Autodesk Inventor part; units mm, degrees
ref_plane "YZ Plane" through (0, 0, 0) normal (1, 0, 0) x (0, 1, 0)
ref_plane "XZ Plane" through (0, 0, 0) normal (0, 1, 0) x (-1, 0, 0)
ref_plane "XY Plane" through (0, 0, 0) normal (0, 0, 1) x (1, 0, 0)
sketch "Esquisse1" plane through (0, 0, 0) normal (0, 0, 1) x (1, 0, 0)
  line L0 (-367.5, -182.5) -> (367.5, -182.5)
  line L1 (367.5, -182.5) -> (367.5, 182.5)
  line L2 (367.5, 182.5) -> (-367.5, 182.5)
  line L3 (-367.5, 182.5) -> (-367.5, -182.5)
  line L4 (-367.5, -182.5) -> (367.5, 182.5) construction
  line L5 (-355, -170) -> (355, -170)
  line L6 (355, -170) -> (355, 170)
  line L7 (355, 170) -> (-355, 170)
  line L8 (-355, 170) -> (-355, -170)
  line L9 (-355, -170) -> (355, 170) construction
  circle A0 centre (-352.5, 167.5) radius 2.5
  circle A1 centre (-352.5, -167.5) radius 2.5
  circle A2 centre (352.5, -167.5) radius 2.5
  circle A3 centre (352.5, 167.5) radius 2.5
  line L10 (-17.5, -40.5) -> (34.5, -40.5)
  line L11 (54.5, -60.5) -> (54.5, -112.5)
  line L12 (34.5, -132.5) -> (-17.5, -132.5)
  line L13 (-37.5, -112.5) -> (-37.5, -60.5)
  line L14 (-37.5, -40.5) -> (54.5, -132.5) construction
  line L15 (54.5, -40.5) -> (-37.5, -132.5) construction
  line L16 (-17.5, -40.5) -> (-37.5, -60.5)
  line L17 (-37.5, -112.5) -> (-17.5, -132.5)
  line L18 (34.5, -132.5) -> (54.5, -112.5)
  line L19 (54.5, -60.5) -> (34.5, -40.5)
  circle A4 centre (-32.75, -45.25) radius 2.2
  circle A5 centre (49.75, -45.25) radius 2.2
  circle A6 centre (49.75, -127.75) radius 2.2
  circle A7 centre (-32.75, -127.75) radius 2.2
  point P0 (0, 0)
  point P1 (-355, -167.5)
  point P2 (-352.5, -170)
  point P3 (352.5, -170)
  point P4 (355, -167.5)
  point P5 (355, 167.5)
  point P6 (352.5, 170)
  point P7 (-355, 167.5)
  point P8 (-352.5, 170)
  point P9 (8.5, -86.5)
  dimension "d0" = 735
  dimension "d1" = 365
  dimension "d2" = 12.5
  dimension "d3" = 12.5
  dimension "d4" = 5
  dimension "d7" = 5
  dimension "d8" = 5
  dimension "d9" = 5
  dimension "d36" = 92
  dimension "d37" = 92
  dimension "d38" = 50
  dimension "d39" = 313
  dimension "d48" = 20
  dimension "d49" = 20
  dimension "d50" = 20
  dimension "d51" = 20
  dimension "d52" = 20
  dimension "d53" = 20
  dimension "d54" = 20
  dimension "d55" = 20
  dimension "d57" = 4.4
  dimension "d58" = 4.4
  dimension "d59" = 4.4
  dimension "d60" = 4.4
  dimension "d61" = 4.75
  dimension "d62" = 4.75
extrude "Extrusion1" add sketch "Esquisse1" along normal blind 2 contours L3 L2 L1 L0 | L8 A1 L5 | A1 L8 A0 L7 A3 L6 A2 L5 | A2 L6 L5 | L8 L7 A0 | A3 L7 L6
properties part number "PlaqueVentilo"
The listing builds one solid part. Answer for the finished solid, in the listing's coordinates (mm). A direction names the side the tool comes from. Round coordinates to 2 decimals unless told otherwise and drop trailing zeros. Loops run counter-clockwise (first coordinate to the right, second up) from the corner with the lowest first, then second, coordinate; pieces in that order, holes last. Notation, with made-up numbers: M 82,-38 L 105,-38 A24 cw 105,-1 Z; hole C 60.25,58 d4. An arc over 180 degrees is marked long. Return JSON: item names as keys, results as strings.
Q1. Find section A-A, the plane x = 18.5. Determine the outline of the cut face in (y, z), plus the area to 3 significant figures.
Results list:
{"outline": "M -182.5,0 L -132.5,0 L -132.5,2 L -182.5,2 Z; M -40.5,0 L 182.5,0 L 182.5,2 L -40.5,2 Z", "area": "546 mm2"}
Q2. Which of the six approach directions +Z, -Z, +X, -X, +Y, -Y give full straight-line access (tool end or side, diameter ignored) to faces 1 (the face through (-5, 3, 0)), 2 (the face through (-28, -122, 1))?
Results list:
{"face 1": "-Z, +X, -X, +Y, -Y", "face 2": "+Z, -Z"}
Q3. Find section B-B, the plane z = 1.4. State how many separate pieces and enclosed holes the cut face has, plus the area to 3 significant figures.
Results list:
{"separate pieces": "1", "enclosed holes": "9", "area": "260,000 mm2"}
Q4. Find the intervals of material crossed by line 1 along X through (y, z) = (-167.5, 1.5); line 2 along Y through (x, z) = (-352.5, 0.5); line 3 along Y through (x, z) = (-32.75, 1.3), in increasing order. Write a range as from..to.
Results list:
{"line 1": "x = -367.5..-355, -350..350, 355..367.5", "line 2": "y = -182.5..-170, -165..165, 170..182.5", "line 3": "y = -182.5..-129.95, -125.55..-117.25, -55.75..-47.45, -43.05..182.5"}
Q5. This flat-tipped pin is pushed along its axis until it touches: pin 1 Ø3.5 at (x, y) = (49.75, -45.25) entering from +Z. Where does it stop, or does it pass through?
Results list:
{"pin 1": "passes through"}
